from build123d import *

# Parameters (mm, degrees)
F0_R     = 25.7
F0_R_2   = 24.85
F1_DEPTH = 7
F2_R     = 27.6
F2_R_2   = 25.7
F3_DEPTH = 12
F5_R     = 37.5
F5_R_2   = 25.7
F6_DEPTH = 4


with BuildPart() as f1:
    # F0 (on Top) → F1 (new body)
    with BuildSketch(Plane.XY):
        Circle(F0_R)
        Circle(F0_R_2, mode=Mode.SUBTRACT)
    extrude(amount=F1_DEPTH)

    # F2 (on Top) → F3 (join)
    with BuildSketch(Plane.XY):
        Circle(F2_R)
        Circle(F2_R_2, mode=Mode.SUBTRACT)
    extrude(amount=F3_DEPTH)

    # F5 (on offset) → F6 (join)
    with BuildSketch(Plane.XY.offset(12)):
        Circle(F5_R)
        Circle(F5_R_2, mode=Mode.SUBTRACT)
    extrude(amount=F6_DEPTH)


solid = f1.part
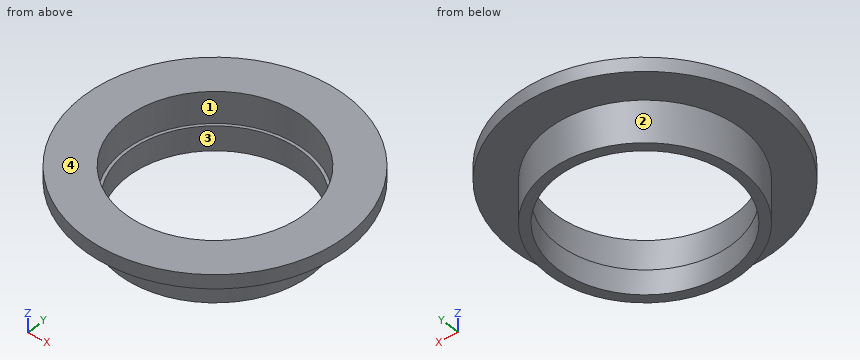
Verification items for the finished model (mm, model axes). Face numbers are marked on the shaded views. Round coordinates to 2 decimals unless told otherwise and drop trailing zeros. Order: outer loops, then holes, each group sorted by start corner. A loop starts at its lowest first (then second) coordinate and runs counter-clockwise, first axis right, second up. Notation, with made-up numbers: (30, 25.25) -> (87, 25.25) arc R29 cw to (87, 53.25) -> close; hole circle Ø8 at (-26.75, 51.5). An arc over 180 degrees is marked (long way). Put each result on its own line as item: value.
1) Section check C-C (z = 5). Record the cut outline in (x, y).
Final values:
outline: circle Ø55.2 at (0, 0); hole circle Ø49.7 at (0, 0)
2) Mould release check, pull along X, two halves, no side actions. Record for the marked faces 1, 2, 3 and 4: +X half, -X half, draft (parallel to the pull), parting line (faces both ways), or undercut.
Final values:
face 1: undercut
face 2: parting line
face 3: undercut
face 4: draft
3) Material ranges on line 1 (Y direction, x = 0, z = 5.25); line 2 (Y direction, x = 0, z = 10.5); line 3 (Z direction, x = 30, y = 20), recorded low to high.
Final values:
line 1: y = -27.6 to -24.85, 24.85 to 27.6
line 2: y = -27.6 to -25.7, 25.7 to 27.6
line 3: z = 12 to 16
4) Depth check by flat-ended pin: pin 1 (5 mm diameter, centred on x = -12.5, y = -29.5, fed in from -Z); pin 2 (3 mm diameter, centred on x = -29.5, y = 26.5, fed in from +Z); pin 3 (1.5 mm diameter, centred on y = 1.5, z = 12.5, fed in from +X); pin 4 (1.5 mm diameter, centred on y = 3, z = 3, fed in from +X). Enter the tip coordinate at first touch or a pass-through.
Final values:
pin 1: stops at z = 12
pin 2: passes through
pin 3: stops at x = 37.49
pin 4: stops at x = 27.51
5) Section check A-A (y = 0). Record the cut outline in (x, z), then the cut area to 3 significant figures.
Final values:
outline: (-37.5, 12) -> (-27.6, 12) -> (-27.6, 0) -> (-24.85, 0) -> (-24.85, 7) -> (-25.7, 7) -> (-25.7, 16) -> (-37.5, 16) -> close; (24.85, 0) -> (27.6, 0) -> (27.6, 12) -> (37.5, 12) -> (37.5, 16) -> (25.7, 16) -> (25.7, 7) -> (24.85, 7) -> close
area: 152 mm^2
6) Section check D-D (z = 10). Record the cut outline in (x, y), then the cut area to 3 significant figures.
Final values:
outline: circle Ø55.2 at (0, 0); hole circle Ø51.4 at (0, 0)
area: 318 mm^2
